Geometry check sheet. Reference: the model listing, model coordinates, mm. Face numbers are marked on the shaded views. A direction names the side the tool comes from. Give positions to 0.01 mm unless a question says otherwise; leave off trailing zeros. Write each loop counter-clockwise with the first axis right and the second up, starting at its lowest first coordinate (ties: lowest second). Pieces come first, ordered by that corner, then holes. Notation, with made-up numbers: M 62.25,30 L 107.25,30 A22 ccw 107.25,66 Z; hole C 40,-16.5 d5. An arc over 180 degrees is marked long. Use one line per item in the form item = value. Start each with the question number.
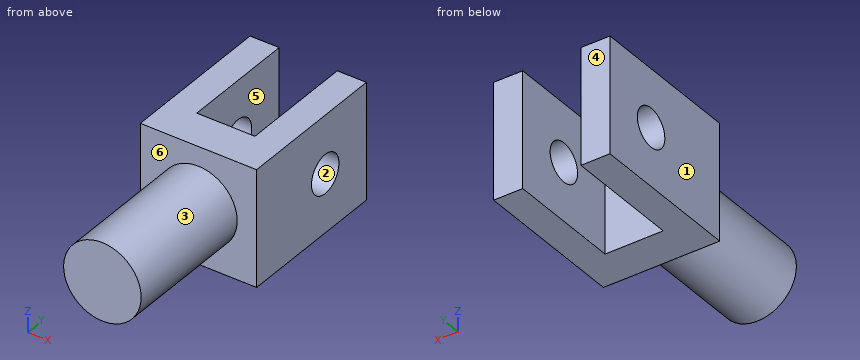
```python
from build123d import *

# Parameters (mm, degrees)
ESQUISSE1_W             = 30
ESQUISSE1_H             = 40
BOSS_EXTRU_1_DEPTH      = 30
ESQUISSE2_W             = 15
ESQUISSE2_H             = 30
ENL_V_MAT_EXTRU_1_DEPTH = 30
ESQUISSE3_R             = 5
ENL_V_MAT_EXTRU_2_DEPTH = 50
ESQUISSE4_R             = 10
BOSS_EXTRU_2_DEPTH      = 35


with BuildPart() as part:
    # Esquisse1 → Boss.-Extru.1 (new body)
    with BuildSketch(Plane.XY):
        with Locations((-15, 20)):
            Rectangle(ESQUISSE1_W, ESQUISSE1_H)
    extrude(amount=BOSS_EXTRU_1_DEPTH)

    # Esquisse2 → Enlèv. mat.-Extru.1 (cut)
    with BuildSketch(Plane.XY.offset(30)):
        with Locations((-15, 25)):
            Rectangle(ESQUISSE2_W, ESQUISSE2_H)
    extrude(amount=-ENL_V_MAT_EXTRU_1_DEPTH, mode=Mode.SUBTRACT)

    # Esquisse3 → Enlèv. mat.-Extru.2 (cut)
    with BuildSketch(Plane.ZY.offset(30)):
        with Locations((15, 25)):
            Circle(ESQUISSE3_R)
    extrude(amount=-ENL_V_MAT_EXTRU_2_DEPTH, mode=Mode.SUBTRACT)

    # Esquisse4 → Boss.-Extru.2 (add)
    with BuildSketch(Plane.XZ):
        with Locations(Location((-15, 15, 0), (0, 0, 90))):  # turned: the seam where the file's is
            Circle(ESQUISSE4_R)
    extrude(amount=BOSS_EXTRU_2_DEPTH)


solid = part.part
```
(1) Depth check by flat-ended pin: pin 1 (1.5 mm diameter, centred on y = -4, z = 26.5, fed in from +X); pin 2 (1.5 mm diameter, centred on y = -10, z = 16, fed in from -X); pin 3 (3 mm diameter, centred on x = -27, z = 15, fed in from -Y); pin 4 (5 mm diameter, centred on x = -12.5, z = 18, fed in from +Y). Enter the tip coordinate at first touch or a pass-through.
(2) Sectioned sample at D-D, the plane x = -15. Record the boundary of the cut face in (y, z), plus the area to 3 significant figures.
(3) Sectioned sample at B-B, the plane z = 17.5. Record the boundary of the cut face in (x, y).
(4) Tool access check on the marked faces 4, 5 and 6. Record the directions out of +Z, -Z, +X, -X, +Y, -Y that give a thin tool (end or side, any length) a straight path to the whole face; none if there is none.
(5) Sectioned sample at C-C, the plane z = 2. Record the boundary of the cut face in (x, y), plus the area to 3 significant figures.
(6) Sectioned sample at A-A, the plane y = 28. Record the boundary of the cut face in (x, z).
(7) Draft check along Z on the marked faces 1, 2 and 3. Enter one of: released by +Z, released by -Z, zero draft, split by the parting line, or undercut.
(8) Thickness scan on probe 1 along Y at (x, z) = (-24.5, 15); probe 2 along X at (y, z) = (25, 28); probe 3 along Y at (x, z) = (-4.5, 15). Record the ranges inside material, lowest first. Write a range as [from, to].
Numbers:
q1.pin_1 = through
q1.pin_2 = -25
q1.pin_3 = 0
q1.pin_4 = 10
q2.outline = M -35,5 L 0,5 L 0,0 L 10,0 L 10,30 L 0,30 L 0,25 L -35,25 Z
q2.area = 1,000 mm2
q3.outline = M -30,0 L -24.68,0 L -24.68,-35 L -5.32,-35 L -5.32,0 L 0,0 L 0,20.67 L -7.5,20.67 L -7.5,10 L -22.5,10 L -22.5,20.67 L -30,20.67 Z; M -30,29.33 L -22.5,29.33 L -22.5,40 L -30,40 Z; M -7.5,29.33 L 0,29.33 L 0,40 L -7.5,40 Z
q4.face_4 = +Z, -Z, +X, -X, +Y
q4.face_5 = +Z, -Z, +Y
q4.face_6 = -Y
q5.outline = M -30,0 L 0,0 L 0,40 L -7.5,40 L -7.5,10 L -22.5,10 L -22.5,40 L -30,40 Z
q5.area = 750 mm2
q6.outline = M -30,0 L -22.5,0 L -22.5,11 L -30,11 Z; M -30,19 L -22.5,19 L -22.5,30 L -30,30 Z; M -7.5,0 L 0,0 L 0,11 L -7.5,11 Z; M -7.5,19 L 0,19 L 0,30 L -7.5,30 Z
q7.face_1 = zero draft
q7.face_2 = undercut
q7.face_3 = split by the parting line
q8.probe_1 = [-35, 20], [30, 40]
q8.probe_2 = [-30, -22.5], [-7.5, 0]
q8.probe_3 = [0, 20], [30, 40]
